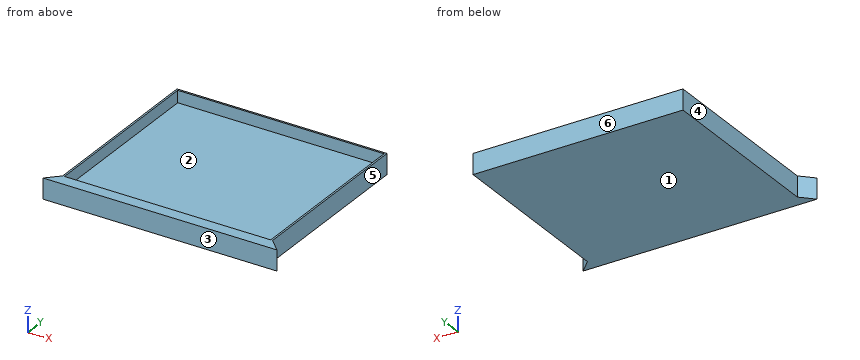
```python
from build123d import *

# Parameters (mm, degrees)
SKETCH_1_W          = 350
SKETCH_1_H          = 320
EXTRUDE_1_DEPTH     = 34
SKETCH_2_W          = 344
SKETCH_2_H          = 314
CUT_EXTRUDE_1_DEPTH = 20
SKETCH_3_W          = 390
SKETCH_3_H          = 34
EXTRUDE_2_DEPTH     = 20
CHAMFER_1_SIZE      = 20


with BuildPart() as part:
    # 草图1 → 凸台-拉伸1 (new body)
    with BuildSketch(Plane.XY):
        Rectangle(SKETCH_1_W, SKETCH_1_H)
    extrude(amount=EXTRUDE_1_DEPTH)

    # 草图2 → 切除-拉伸1 (cut)
    with BuildSketch(Plane.XY.offset(34)):
        Rectangle(SKETCH_2_W, SKETCH_2_H)
    extrude(amount=-CUT_EXTRUDE_1_DEPTH, mode=Mode.SUBTRACT)

    # 草图3 → 凸台-拉伸2 (add)
    with BuildSketch(Plane.XZ.offset(160)):
        with Locations((0, 17)):
            Rectangle(SKETCH_3_W, SKETCH_3_H)
    extrude(amount=-EXTRUDE_2_DEPTH)

    # 倒角1
    chamfer_1_edges = [part.edges().sort_by_distance(p)[0] for p in [
        (195, -140, 17),
        (-195, -140, 17),
    ]]
    chamfer(chamfer_1_edges, length=CHAMFER_1_SIZE - 0.0001)  # a hair under: the kernel refuses the full size


solid = part.part
```
CAD build for the part. Positions are in the model's coordinates, mm. Face numbers are marked on the shaded views. A direction names the side the tool comes from. Coordinates: 2 decimals unless noted, no trailing zeros. Loops run counter-clockwise (first coordinate to the right, second up) from the corner with the lowest first, then second, coordinate; pieces in that order, holes last. Notation, with made-up numbers: (29, -3.75) - (79, -3.75) arc R27 ccw to (79, 29.25) - close; hole circle Ø2 at (36.25, -24). An arc over 180 degrees is marked (long way). Return JSON: item names as keys, results as strings.
1. 3-axis set-ups, long thin cutter, end or side, ignore diameter. For the marked faces 4, 5 and 6: which of +Z, -Z, +X, -X, +Y, -Y reach the whole face in a straight line?
Result:
{"face 4": "+Z, -Z, -X, +Y", "face 5": "+Z, -Z, +X, +Y", "face 6": "+Z, -Z, +X, -X, +Y"}
2. Mould opens along Y. For the marked faces 1, 2 and 3 say: released by +Y, released by -Y, zero draft, split by the parting line, or undercut.
Result:
{"face 1": "zero draft", "face 2": "undercut", "face 3": "released by -Y"}
3. Drop flat-ended pins along their axis: pin 1 (6 mm diameter, centred on y = 58, z = 29, fed in from +X); pin 2 (6 mm diameter, centred on y = -110, z = 11.5, fed in from -X); pin 3 (12 mm diameter, centred on x = 11.5, y = 16, fed in from +Z). Give the stop position or say it passes through.
Result:
{"pin 1": "stops at x = 175", "pin 2": "stops at x = -175", "pin 3": "stops at z = 14"}
4. Band-saw the part on B-B (x = 26). Give the cut face in (y, z).
Result:
{"outline": "(-160, 0) - (160, 0) - (160, 34) - (157, 34) - (157, 14) - (-140, 14) - (-140, 34) - (-160, 34) - close"}
5. Probe L1, parallel to X at y = 103, z = 22; L2, parallel to Y at x = -1, z = 33; L3, parallel to X at y = 56.5, z = 8. List the from-to ranges inside material, lowest first. Write a range as from..to.
Result:
{"L1": "x = -175..-172, 172..175", "L2": "y = -160..-140, 157..160", "L3": "x = -175..175"}
6. Band-saw the part on D-D (y = 68). Give the cut face in (x, z), and give its area (3 significant figures).
Result:
{"outline": "(-175, 0) - (175, 0) - (175, 34) - (172, 34) - (172, 14) - (-172, 14) - (-172, 34) - (-175, 34) - close", "area": "5,020 mm2"}
